Design review of the part built by this model. Coordinates are the model's own, in mm. Face numbers are marked on the shaded views. A direction names the side the tool comes from. Give positions to 0.01 mm unless a question says otherwise; leave off trailing zeros. Write each loop counter-clockwise with the first axis right and the second up, starting at its lowest first coordinate (ties: lowest second). Pieces come first, ordered by that corner, then holes. Notation, with made-up numbers: M -7.5,16.25 L 1.5,16.25 A34 cw 1.5,46.25 Z; hole C 65,-0.5 d8. An arc over 180 degrees is marked long. Use one line per item in the form item = value. Start each with the question number.
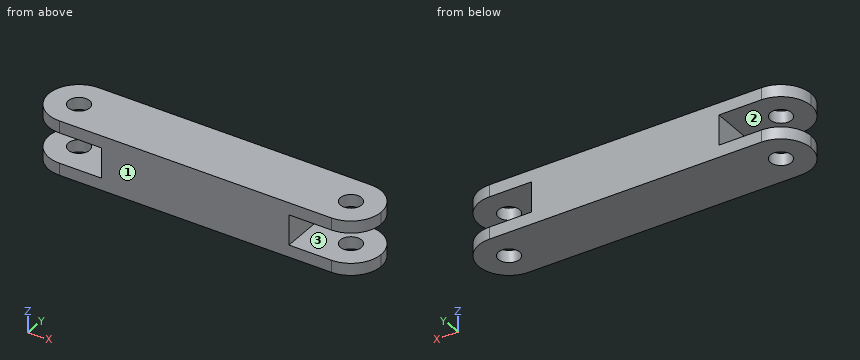
from build123d import *

# Parameters (mm, degrees)
SKETCH_5_W               = 55
SKETCH_5_H               = 9
EXTRUDE_1_DEPTH          = 10
FILLET_2_R               = 5
CUT_EXTRUDE_1_REACH      = 58.622
SKETCH_6_R               = 1.75
CUT_EXTRUDE_4_DEPTH      = 57.621550668
CUT_EXTRUDE_4_DEPTH_BACK = 57.621550668
SKETCH_7_W               = 12
SKETCH_7_H               = 5


with BuildPart() as part:
    # 草图5 → 凸台-拉伸1 (new body)
    with BuildSketch(Plane(origin=(0, 0, 0), x_dir=(1, 0, 0), z_dir=(0, 1, 0))):
        with Locations((27.5, -4.5)):
            Rectangle(SKETCH_5_W, SKETCH_5_H)
    extrude(amount=EXTRUDE_1_DEPTH)

    # 圆角2
    fillet_2_edges = [part.edges().sort_by_distance(p)[0] for p in [
        (55, 0, 4.5),
        (55, 10, 4.5),
        (0, 0, 4.5),
        (0, 10, 4.5),
    ]]
    fillet(fillet_2_edges, radius=FILLET_2_R - 0.0001)  # a hair under: the kernel refuses the full size

    # 草图6 → 切除-拉伸1 (cut, up to next)
    with BuildSketch(Plane.XY.offset(9), mode=Mode.PRIVATE) as cut_extrude_1_sk1:
        with Locations((5, 5)):
            Circle(SKETCH_6_R)
    cut_extrude_1_tool1 = extrude(cut_extrude_1_sk1.sketch, amount=-CUT_EXTRUDE_1_REACH, mode=Mode.PRIVATE) & part.part
    # 草图6 → 切除-拉伸1 (cut, up to next)
    with BuildSketch(Plane.XY.offset(9), mode=Mode.PRIVATE) as cut_extrude_1_sk2:
        with Locations((50, 5)):
            Circle(SKETCH_6_R)
    cut_extrude_1_tool2 = extrude(cut_extrude_1_sk2.sketch, amount=-CUT_EXTRUDE_1_REACH, mode=Mode.PRIVATE) & part.part
    add(cut_extrude_1_tool1.solids().sort_by_distance((5, 5, 9))[0], mode=Mode.SUBTRACT)
    add(cut_extrude_1_tool2.solids().sort_by_distance((50, 5, 9))[0], mode=Mode.SUBTRACT)

    # 草图7 → 切除-拉伸4 (cut, two sides: drawn at the far end of the back side and taken through both)
    with BuildSketch(Plane(origin=(0, 0, 0), x_dir=(1, 0, 0), z_dir=(0, 1, 0)).offset(-CUT_EXTRUDE_4_DEPTH_BACK)):
        with Locations((6, -4.5)):
            Rectangle(SKETCH_7_W, SKETCH_7_H)
        with Locations((49, -4.5)):
            Rectangle(SKETCH_7_W, SKETCH_7_H)
    extrude(amount=CUT_EXTRUDE_4_DEPTH + CUT_EXTRUDE_4_DEPTH_BACK, mode=Mode.SUBTRACT)


solid = part.part
1. We need section C-C (y = 4). State the section outline as (x, z) points.
2. We need section D-D (z = 5.5). State the section outline as (x, y) points.
3. To check wall thickness, follow L1, parallel to Z at x = 7, y = 6.25; L2, parallel to Y at x = 5, z = 7.45; L3, parallel to X at y = 4.25, z = 1.75. State the ranges of each line that lie inside material, in increasing order.
4. For the marked faces 1, 2 and 3, list the 3-axis set-ups (+Z, -Z, +X, -X, +Y, -Y) from which the entire face can be reached by the end or side of a thin tool; tool diameter is ignored.
5. We need section B-B (z = 1). Give the number of separate pieces and of enclosed holes in the cut face, and give its area (3 significant figures).
6. Clearance check with flat-ended pins moving along their axes: pin 1 Ø4 at (y, z) = (5, 4.5) entering from +X; pin 2 Ø2.5 at (y, z) = (7.5, 4) entering from -X. State where each tip first meets the part, or that it passes through.
7. We need section A-A (x = 10). State the section outline as (y, z) points, and give its area (3 significant figures).
Answer block:
q1.outline = M 0.1,0 L 3.56,0 L 3.56,2 L 0.1,2 Z; M 0.1,7 L 3.56,7 L 3.56,9 L 0.1,9 Z; M 6.44,0 L 48.56,0 L 48.56,2 L 43,2 L 43,7 L 48.56,7 L 48.56,9 L 6.44,9 L 6.44,7 L 12,7 L 12,2 L 6.44,2 Z; M 51.44,0 L 54.9,0 L 54.9,2 L 51.44,2 Z; M 51.44,7 L 54.9,7 L 54.9,9 L 51.44,9 Z
q2.outline = M 12,0 L 43,0 L 43,10 L 12,10 Z
q3.L1 = 0 to 2, 7 to 9
q3.L2 = 0 to 3.25, 6.75 to 10
q3.L3 = 0.06 to 3.42, 6.58 to 48.42, 51.58 to 54.94
q4.face_1 = +Z, -Z, +X, -X, -Y
q4.face_2 = -X, +Y, -Y
q4.face_3 = +X, +Y, -Y
q5.separate_pieces = 1
q5.enclosed_holes = 2
q5.area = 509 mm^2
q6.pin_1 = 43
q6.pin_2 = 12
q7.outline = M 0,0 L 10,0 L 10,2 L 0,2 Z; M 0,7 L 10,7 L 10,9 L 0,9 Z
q7.area = 40.0 mm^2
